The model under review builds one solid part; all positions refer to its coordinate system, in mm. A direction names the side the tool comes from. Coordinates: 2 decimals unless noted, no trailing zeros. Order: outer loops, then holes, each group sorted by start corner. A loop starts at its lowest first (then second) coordinate and runs counter-clockwise, first axis right, second up. Notation, with made-up numbers: (80, -15) -> (85, -15) arc R22 cw to (85, 24) -> close; hole circle Ø8 at (-4.5, -16). An arc over 180 degrees is marked (long way). Use one line per item in the form item = value. Start each with the question number.
(1) Insertion check: pin 1 Ø1.5 at (y, z) = (0, 9.5) entering from +X; pin 2 Ø2.5 at (x, z) = (9, 4) entering from -Y; pin 3 Ø8 at (y, z) = (12.5, 8.5) entering from -X; pin 4 Ø12 at (x, y) = (78, -22.5) entering from -Z. Each pin has a flat end and moves straight along its axis. Give the tip position at first contact, or say it passes through.
(2) Take a section at B-B (x = 37). State the section outline as (y, z) points.
(3) Mouldability with a two-part tool opening along Z and no side actions: class faces 6 (the cylindrical face through (-10.9, 4.43, 8.71)), 7 (the cylindrical face through (0.12, -6.35, 7.51)), 8 (the cylindrical face through (-10.6, -8.66, 7.36)), 9 (the flat face through (55, 0, 0)) as +Z half, -Z half, draft (parallel to the pull), parting line (faces both ways), or undercut.
(4) Take a section at A-A (z = 12.5). State the section outline as (x, y) points (3 decimals), then the cut area to 3 significant figures.
(5) Wall thickness on line 1 along X through (y, z) = (3.25, 7.62); line 2 along X through (y, z) = (-5, 6.5); line 3 along Y through (x, z) = (81, 9.5): over which ranges is each line inside the solid? List them lowest first.
(6) For faces 1 (the flat face through (101.6, -20, 8)), 2 (the flat face through (-10, 7.679, 8)), 3 (the flat face through (101.6, 21, 8)), 4 (the flat face through (9, -1.27, 8)), 5 (the cylindrical face through (-0.12, 6.35, 7.51)), list the 3-axis set-ups (+Z, -Z, +X, -X, +Y, -Y) from which the entire face can be reached by the end or side of a thin tool; tool diameter is ignored.
(7) Take a section at C-C (y = 20.5). State the section outline as (x, z) points.
```python
from build123d import *

# Parameters (mm, degrees)
BOSS_EXTRUDE1_DEPTH     = 15.24
CUT_EXTRUDE1_DEPTH      = 136.965704146
CUT_EXTRUDE1_DEPTH_BACK = 136.965704146
SKETCH2_R               = 2.032
SKETCH3_W               = 13.96136878
SKETCH3_H               = 14.958609408
CUT_EXTRUDE2_DEPTH      = 136.965704158


with BuildPart() as part:
    # Sketch1 → Boss-Extrude1 (new body)
    with BuildSketch(Plane.XY):
        with BuildLine():
            Line((14.199031657, -12.7), (101.6, -12.7))
            Line((101.6, -12.7), (101.6, -28.448))
            Line((101.6, -28.448), (132.08, 0))
            Line((132.08, 0), (101.6, 28.448))
            Line((101.6, 28.448), (101.6, 12.7))
            Line((101.6, 12.7), (14.199031657, 12.7))
            ThreePointArc((14.199031657, 12.7), (-6.20014954, 18.012791168), (-19.007619525, 1.27))
            Line((-19.007619525, 1.27), (-6.221703947, 1.27))
            ThreePointArc((-6.221703947, 1.27), (0, 6.35), (6.221703947, 1.27))
            Line((6.221703947, 1.27), (11.289096091, 1.27))
            ThreePointArc((11.289096091, 1.27), (17.374031657, 0), (11.289096091, -1.27))
            Line((11.289096091, -1.27), (6.221703947, -1.27))
            ThreePointArc((6.221703947, -1.27), (0, -6.35), (-6.221703947, -1.27))
            Line((-6.221703947, -1.27), (-19.007619525, -1.27))
            ThreePointArc((-19.007619525, -1.27), (-6.20014954, -18.012791168), (14.199031657, -12.7))
        make_face()
    extrude(amount=BOSS_EXTRUDE1_DEPTH)

    # Sketch2 → Cut-Extrude1 (cut, two sides: drawn at the far end of the back side and taken through both)
    with BuildSketch(Plane(origin=(0, 0, 0), x_dir=(1, 0, 0), z_dir=(0, 1, 0)).offset(-CUT_EXTRUDE1_DEPTH_BACK)):
        with Locations(Location((-12.614661736, -7.62, 0), (0, 0, 270))):
            Circle(SKETCH2_R)
    extrude(amount=CUT_EXTRUDE1_DEPTH + CUT_EXTRUDE1_DEPTH_BACK, mode=Mode.SUBTRACT)

    # Sketch3 → Cut-Extrude2 (cut, through all)
    with BuildSketch(Plane.XY.offset(15.24)):
        with Locations((-14.567066479, 15.158057533)):
            Rectangle(SKETCH3_W, SKETCH3_H)
    extrude(amount=-CUT_EXTRUDE2_DEPTH, mode=Mode.SUBTRACT)


solid = part.part
```
Findings:
q1.pin_1 = 132.08
q1.pin_2 = -17.4
q1.pin_3 = -7.59
q1.pin_4 = through
q2.outline = (-12.7, 0) -> (12.7, 0) -> (12.7, 15.24) -> (-12.7, 15.24) -> close
q3.face_6 = undercut
q3.face_7 = draft
q3.face_8 = undercut
q3.face_9 = -Z half
q4.outline = (-19.008, -1.27) arc R19.05 ccw to (14.199, -12.7) -> (101.6, -12.7) -> (101.6, -28.448) -> (132.08, 0) -> (101.6, 28.448) -> (101.6, 12.7) -> (14.199, 12.7) arc R19.05 ccw to (-7.586, 17.474) -> (-7.586, 7.679) -> (-17.434, 7.679) arc R19.05 ccw to (-19.008, 1.27) -> (-6.222, 1.27) arc R6.35 cw to (6.222, 1.27) -> (11.289, 1.27) arc R3.175 cw (long way) to (11.289, -1.27) -> (6.222, -1.27) arc R6.35 cw to (-6.222, -1.27) -> close
q4.area = 3,880 mm²
q5.line_1 = -18.77 to -14.65, -10.58 to -5.46, 5.46 to 128.6
q5.line_2 = -18.38 to -14.31, -10.92 to -3.91, 3.91 to 126.72
q5.line_3 = -12.7 to 12.7
q6.face_1 = +Z, -Z, -Y
q6.face_2 = +Z, -Z, -X, +Y
q6.face_3 = +Z, -Z, +Y
q6.face_4 = +Z, -Z, -X
q6.face_5 = +Z, -Z
q7.outline = (101.6, 0) -> (110.12, 0) -> (110.12, 15.24) -> (101.6, 15.24) -> close
